The model under review builds one solid part; all positions refer to its coordinate system, in mm. Round coordinates to 2 decimals unless told otherwise and drop trailing zeros. Order: outer loops, then holes, each group sorted by start corner. A loop starts at its lowest first (then second) coordinate and runs counter-clockwise, first axis right, second up. Notation, with made-up numbers: M -3,73 L 26,73 A28 ccw 26,93 Z; hole C 87,11 d10. An arc over 180 degrees is marked long. Answer as a JSON object with one key per item and string values. Group by question number.
1) Consider section C-C, the plane x = 87.5. Write out the cut boundary in (y, z).
2) The part is to be moulded in two halves that separate along X. For faces 1 (the cylindrical face through (1.2, 143, 6.6)), 2 (the cylindrical face through (1.65, 141.99, 2.71)), 3 (the cylindrical face through (-1.84, 143.99, 3.82)), 4 (the flat face through (9, 143, 0)), say which applies: +X half, -X half, draft (parallel to the pull), parting line (faces both ways), or undercut.
3) Insertion check: pin 1 Ø1 at (x, z) = (19, 4.5) entering from +Y; pin 2 Ø1 at (y, z) = (109, 2.5) entering from +X; pin 3 Ø5 at (x, z) = (42.5, 4) entering from -Y. Each pin has a flat end and moves straight along its axis. Give the tip position at first contact, or say it passes through.
4) Consider section B-B, the plane y = 98.5. Write out the cut boundary in (x, z).
5) Consider section D-D, the plane x = 61.5. Write out the cut boundary in (y, z).
6) To check wall thickness, follow line 1 (X direction, y = 113.5, z = 5.75); line 2 (X direction, y = 127.5, z = 5.25); line 3 (Y direction, x = -75.5, z = 1.25). State the ranges of each line that lie inside material, in increasing order.
7) Consider section A-A, the plane x = 0. Write out the cut boundary in (y, z), then the cut area to 3 significant figures.
```python
from build123d import *

# Parameters (mm, degrees)
BOSS_EXTRU_1_DEPTH           = 10
ENL_V_MAT_EXTRU_1_REACH      = 183.602
ENL_V_MAT_EXTRU_1_END_RADIUS = 144
ESQUISSE3_R                  = 2


with BuildPart() as part:
    # Esquisse2 → Boss.-Extru.1 (new body)
    with BuildSketch(Plane.XY):
        with BuildLine():
            Line((-108.89070765, 91.141723636), (-110.196113775, 92.697446075))
            ThreePointArc((-110.196113775, 92.697446075), (-0.087455631, 143.999973443), (110.083436481, 92.831228649))
            Line((110.083436481, 92.831228649), (108.778310923, 91.275840575))
            ThreePointArc((108.778310923, 91.275840575), (-0.087493397, 141.999973045), (-108.89070765, 91.141723636))
        make_face()
    extrude(amount=BOSS_EXTRU_1_DEPTH)

    # Enlèv. mat.-Extru.1: up to this cylinder (the profile starts inside it)
    enl_v_mat_extru_1_end = Plane(origin=(0, 0, 5), z_dir=(0, 0, -1)) * Cylinder(ENL_V_MAT_EXTRU_1_END_RADIUS, 656.204, mode=Mode.PRIVATE)
    # Esquisse3 → Enlèv. mat.-Extru.1 (cut, up to the surface)
    with BuildSketch(Plane(origin=(0, 0, 0), x_dir=(1, 0, 0), z_dir=(0, 1, 0)), mode=Mode.PRIVATE) as enl_v_mat_extru_1_sk1:
        with Locations(Location((0, -5, 0), (0, 0, 90))):
            Circle(ESQUISSE3_R)
    enl_v_mat_extru_1_tool1 = extrude(enl_v_mat_extru_1_sk1.sketch, amount=ENL_V_MAT_EXTRU_1_REACH, mode=Mode.PRIVATE) & enl_v_mat_extru_1_end
    add(enl_v_mat_extru_1_tool1.solids().sort_by_distance((0, 0, 5))[0], mode=Mode.SUBTRACT)


solid = part.part
```
Results list:
{
 "1": {"outline": "M 111.84,0 L 114.37,0 L 114.37,10 L 111.84,10 Z"},
 "2": {"face 1": "undercut", "face 2": "undercut", "face 3": "parting line", "face 4": "draft"},
 "3": {"pin 1": "y = 142.81", "pin 2": "x = 94.68", "pin 3": "y = 134.68"},
 "4": {"outline": "M -105.04,0 L -102.28,0 L -102.28,10 L -105.04,10 Z; M 102.28,0 L 105.04,0 L 105.04,10 L 102.28,10 Z"},
 "5": {"outline": "M 127.99,0 L 130.21,0 L 130.21,10 L 127.99,10 Z"},
 "6": {"line 1": "-88.62 to -85.33, 85.33 to 88.62", "line 2": "-66.93 to -62.51, 62.51 to 66.93", "line 3": "120.27 to 122.62"},
 "7": {"outline": "M 142,0 L 144,0 L 144,3 L 142,3 Z; M 142,7 L 144,7 L 144,10 L 142,10 Z", "area": "12.0 mm^2"}
}
